Work out the finished part from the listing and answer in its coordinate system (mm). A direction names the side the tool comes from. Coordinates: 2 decimals unless noted, no trailing zeros. Write each loop counter-clockwise with the first axis right and the second up, starting at its lowest first coordinate (ties: lowest second). Pieces come first, ordered by that corner, then holes. Notation, with made-up numbers: (-14, 10.25) - (13, 10.25) arc R16 ccw to (13, 26.25) - close; hole circle Ø7 at (-26.5, 19.5). An arc over 180 degrees is marked (long way). Use one line per item in the form item = value. Start each with the question number.
Item 1: Determine the mould class of faces 1 (the flat face through (-37, -63, 2)), 2 (the flat face through (100, -1, 2)), 3 (the flat face through (-1, 1, 5)) for opening direction X: released by +X, released by -X, zero draft, split by the parting line, or undercut.
Item 2: A cutting plane is placed at B-B (y = -60). Write down the section's boundary in (x, z), then the cut area to 3 significant figures.
Item 3: A cutting plane is placed at A-A (x = -90). Write down the section's boundary in (y, z).
Item 4: For faces 4 (the flat face through (-37, -66, 2)), 5 (the cylindrical face through (99, 73, 2)), determine the directions among +Z, -Z, +X, -X, +Y, -Y from which every point of the face is accessible in a straight line to the end or side of a thin tool.
Item 5: Consider probe 1 along Y at (x, z) = (58, 4.05); probe 2 along Y at (x, z) = (-90, 1.3); probe 3 along X at (y, z) = (-57.5, 3.35). Determine where each line is inside the solid, lowest interval first.
Item 6: A cutting plane is placed at C-C (x = -47). Write down the section's boundary in (y, z), then the cut area to 3 significant figures.
from build123d import *

# Parameters (mm, degrees)
F0_R     = 3
F0_W     = 6
F0_H     = 3
F1_DEPTH = 5


with BuildPart() as f1:
    # F0 (on Top) → F1 (new body)
    with BuildSketch(Plane.XY):
        with BuildLine():
            ThreePointArc((100, 70), (98.535534, 73.535534), (95, 75))
            Line((95, 75), (-95, 75))
            ThreePointArc((-95, 75), (-98.535534, 73.535534), (-100, 70))
            Line((-100, 70), (-100, -70))
            ThreePointArc((-100, -70), (-98.535534, -73.535534), (-95, -75))
            Line((-95, -75), (95, -75))
            ThreePointArc((95, -75), (98.535534, -73.535534), (100, -70))
            Line((100, -70), (100, 70))
        make_face()
        with Locations((-90, -60)):
            Circle(F0_R, mode=Mode.SUBTRACT)
        with Locations((-47, -60)):
            Circle(F0_R, mode=Mode.SUBTRACT)
        with Locations((-37, -64.5)):
            Rectangle(F0_W, F0_H, mode=Mode.SUBTRACT)
        with Locations((-37, -55.5)):
            Rectangle(F0_W, F0_H, mode=Mode.SUBTRACT)
        with Locations((37, -64.5)):
            Rectangle(F0_W, F0_H, mode=Mode.SUBTRACT)
        with Locations((47, -60)):
            Circle(F0_R, mode=Mode.SUBTRACT)
        with Locations((37, -55.5)):
            Rectangle(F0_W, F0_H, mode=Mode.SUBTRACT)
        with Locations((90, -60)):
            Circle(F0_R, mode=Mode.SUBTRACT)
        with Locations((-60, 55.5)):
            Rectangle(F0_W, F0_H, mode=Mode.SUBTRACT)
        with Locations((-90, 60)):
            Circle(F0_R, mode=Mode.SUBTRACT)
        with Locations((-70, 60)):
            Circle(F0_R, mode=Mode.SUBTRACT)
        with Locations((-60, 64.5)):
            Rectangle(F0_W, F0_H, mode=Mode.SUBTRACT)
        with Locations((60, 55.5)):
            Rectangle(F0_W, F0_H, mode=Mode.SUBTRACT)
        with Locations((60, 64.5)):
            Rectangle(F0_W, F0_H, mode=Mode.SUBTRACT)
        with Locations((70, 60)):
            Circle(F0_R, mode=Mode.SUBTRACT)
        with Locations((90, 60)):
            Circle(F0_R, mode=Mode.SUBTRACT)
    extrude(amount=F1_DEPTH)


solid = f1.part
Answer:
q1.face_1 = undercut
q1.face_2 = released by +X
q1.face_3 = zero draft
q2.outline = (-100, 0) - (-93, 0) - (-93, 5) - (-100, 5) - close; (-87, 0) - (-50, 0) - (-50, 5) - (-87, 5) - close; (-44, 0) - (44, 0) - (44, 5) - (-44, 5) - close; (50, 0) - (87, 0) - (87, 5) - (50, 5) - close; (93, 0) - (100, 0) - (100, 5) - (93, 5) - close
q2.area = 880 mm²
q3.outline = (-75, 0) - (-63, 0) - (-63, 5) - (-75, 5) - close; (-57, 0) - (57, 0) - (57, 5) - (-57, 5) - close; (63, 0) - (75, 0) - (75, 5) - (63, 5) - close
q4.face_4 = +Z, -Z
q4.face_5 = +Z, -Z, +X, +Y
q5.probe_1 = -75 to 54, 57 to 63, 66 to 75
q5.probe_2 = -75 to -63, -57 to 57, 63 to 75
q5.probe_3 = -100 to -91.66, -88.34 to -48.66, -45.34 to 45.34, 48.66 to 88.34, 91.66 to 100
q6.outline = (-75, 0) - (-63, 0) - (-63, 5) - (-75, 5) - close; (-57, 0) - (75, 0) - (75, 5) - (-57, 5) - close
q6.area = 720 mm²
